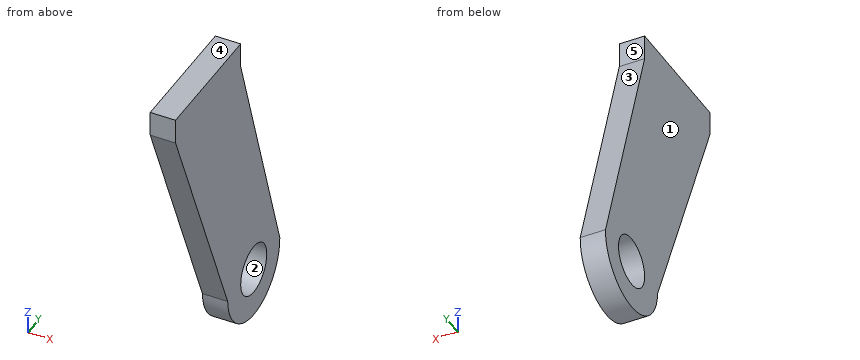
from build123d import *

# Parameters (mm, degrees)
SKETCH1_R           = 2
BOSS_EXTRUDE1_DEPTH = 2


with BuildPart() as part:
    # Sketch1 → Boss-Extrude1 (new body)
    with BuildSketch(Plane(origin=(0, 0, 0), x_dir=(0, 0, -1), z_dir=(1, 0, 0))):
        with BuildLine():
            Line((-0.003608009, 4.426390949), (19.120298853, 10.431566954))
            ThreePointArc((19.120298853, 10.431566954), (23.223332093, 6.557543739), (19.369494044, 2.435545445))
            Line((19.369494044, 2.435545445), (-0.003608009, -5.573609051))
            Line((-0.003608009, -5.573609051), (-2.003608009, -5.573609051))
            Line((-2.003608009, -5.573609051), (-2.003608009, 4.426390949))
            Line((-2.003608009, 4.426390949), (-0.003608009, 4.426390949))
        make_face()
        with Locations((19.225273181, 6.432944643)):
            Circle(SKETCH1_R, mode=Mode.SUBTRACT)
    extrude(amount=BOSS_EXTRUDE1_DEPTH)


solid = part.part
Can you work these out from the model? Positions are in its coordinate system, mm. Face numbers are marked on the shaded views. A direction names the side the tool comes from. Coordinates: 2 decimals unless noted, no trailing zeros. Write each loop counter-clockwise with the first axis right and the second up, starting at its lowest first coordinate (ties: lowest second). Pieces come first, ordered by that corner, then holes. Notation, with made-up numbers: (52, 56.25) -> (108, 56.25) arc R12 ccw to (108, 78.25) -> close; hole circle Ø4 at (63.25, 87.5). An arc over 180 degrees is marked (long way). Write each question's results on one line, items separated by ' | '. Start each with the question number.
Item 1: If we section it at B-B, the plane y = 5.75: Write out the boundary of the cut face in (x, z), and give its area (3 significant figures).
Item 2: If we section it at C-C, the plane x = 1: Write out the boundary of the cut face in (y, z).
Item 3: If we section it at D-D, the plane y = 3.75: Write out the boundary of the cut face in (x, z).
Item 4: Please list where these lines run through material, in increasing order: probe 1 along Y at (x, z) = (0.1, -18); probe 2 along Y at (x, z) = (1.7, 0.5); probe 3 along Y at (x, z) = (1.4, -7.25).
Item 5: If we section it at A-A, the plane z = -18.25: Write out the boundary of the cut face in (x, y), and give its area (3 significant figures).
Item 6: On a 3-axis mill with a long thin cutter (end or side, diameter ignored), from which of +Z, -Z, +X, -X, +Y, -Y can I reach the whole of each face in a straight line? I mean the marked faces 4 and 5. Say none if no direction works.
Item 7: Thinking about a two-plate mould opening in Z: for the marked faces 1, 2 and 3, which applies, released by +Z, released by -Z, zero draft, split by the parting line, or undercut?
Answer block:
1) outline: (0, -23.17) -> (2, -23.17) -> (2, -21.11) -> (0, -21.11) -> close; (0, -17.35) -> (2, -17.35) -> (2, -4.21) -> (0, -4.21) -> close | area: 30.4 mm²
2) outline: (-5.57, 0) -> (2.44, -19.37) arc R4 ccw to (10.43, -19.12) -> (4.43, 0) -> (4.43, 2) -> (-5.57, 2) -> close; hole circle Ø4 at (6.43, -19.23)
3) outline: (0, -22.19) -> (2, -22.19) -> (2, 2) -> (0, 2) -> close
4) probe 1: 1.87 to 4.85, 8.01 to 10.08 | probe 2: -5.57 to 4.43 | probe 3: -2.57 to 6.7
5) outline: (0, 1.97) -> (2, 1.97) -> (2, 4.69) -> (0, 4.69) -> close; (0, 8.18) -> (2, 8.18) -> (2, 10.16) -> (0, 10.16) -> close | area: 9.39 mm²
6) face 4: +Z, +X, -X, +Y, -Y | face 5: +Z, +X, -X, +Y
7) face 1: zero draft | face 2: undercut | face 3: released by +Z
